Source: CAD feature listing. Evaluate the final solid. Frame: model axes, mm. A direction names the side the tool comes from. Round coordinates to 2 decimals unless told otherwise and drop trailing zeros. Loops run counter-clockwise (first coordinate to the right, second up) from the corner with the lowest first, then second, coordinate; pieces in that order, holes last. Notation, with made-up numbers: (13, 81) - (61, 81) arc R29 cw to (61, 112) - close; hole circle Ø11 at (-30, 53). An arc over 180 degrees is marked (long way). Write item = value, one per line. Start each with the question number.
from build123d import *

# Parameters (mm, degrees)
SKETCH1_R           = 2.5
BOSS_EXTRUDE1_DEPTH = 10
SKETCH2_R           = 7.5
BOSS_EXTRUDE2_DEPTH = 60
SKETCH3_R           = 2.5
CUT_EXTRUDE1_DEPTH  = 15


with BuildPart() as part:
    # Sketch1 → Boss-Extrude1 (new body)
    with BuildSketch(Plane.XY):
        with BuildLine():
            Line((2.5, 0), (37.6, 0))
            ThreePointArc((37.6, 0), (39.367766953, 0.732233047), (40.1, 2.5))
            Line((40.1, 2.5), (40.1, 37.6))
            ThreePointArc((40.1, 37.6), (39.367766953, 39.367766953), (37.6, 40.1))
            Line((37.6, 40.1), (2.5, 40.1))
            ThreePointArc((2.5, 40.1), (0.732233047, 39.367766953), (0, 37.6))
            Line((0, 37.6), (0, 2.5))
            ThreePointArc((0, 2.5), (0.732233047, 0.732233047), (2.5, 0))
        make_face()
        with Locations((6.75, 33.35)):
            Circle(SKETCH1_R, mode=Mode.SUBTRACT)
        with Locations((33.35, 6.75)):
            Circle(SKETCH1_R, mode=Mode.SUBTRACT)
    extrude(amount=BOSS_EXTRUDE1_DEPTH)

    # Sketch2 → Boss-Extrude2 (add)
    with BuildSketch(Plane.XY.offset(10)):
        with Locations((20.05, 20.05)):
            Circle(SKETCH2_R)
    extrude(amount=BOSS_EXTRUDE2_DEPTH)

    # Sketch3 → Cut-Extrude1 (cut)
    with BuildSketch(Plane.XY.offset(70)):
        with Locations((20.05, 20.05)):
            Circle(SKETCH3_R)
    extrude(amount=-CUT_EXTRUDE1_DEPTH, mode=Mode.SUBTRACT)


solid = part.part
(1) Cut plane C-C (z = 7). Output: boundary loops of the cut face in (x, y), and give its area (3 significant figures).
(2) Access query for faces 1 (the face through (29, 20, 10)), 2 (the face through (39.387, 39.348, 4.93)). Directions: +Z, -Z, +X, -X, +Y, -Y. A direction counts if a zero-diameter tool reaches every point of the face in a straight line with its end or side. Return the directions, or none.
(3) Cut plane D-D (x = 20.05). Output: boundary loops of the cut face in (y, z), and give its area (3 significant figures).
(4) Mould query, pull axis Y, two halves, no side actions, for faces 3 (the face through (26.98, 17.18, 39.58)), 4 (the face through (20, 20, 55)), 5 (the face through (0, 20, 5)), 6 (the face through (21.2, 17.83, 62.6)). Classes: +Y half, -Y half, draft (parallel to the pull), parting line (faces both ways), or undercut.
(5) Pin query (flat end, axial travel): P1, Ø1, axis at y = 18.5, z = 44, coming from the +X side; P2, Ø6, axis at y = 15, z = 62.5, coming from the -X side; P3, Ø8, axis at y = 18.5, z = 47.5, coming from the -X side. Return the tip coordinate at first contact, or that it passes through.
(6) Cut plane A-A (y = 33.35). Output: boundary loops of the cut face in (x, z).
(7) Cut plane B-B (x = 6.75). Output: boundary loops of the cut face in (y, z).
(8) Material intervals for line 1 along Y through (x, z) = (20, 60); line 2 along Y through (x, z) = (33.35, 3), sorted ascending. Write a range as from..to.
Solution:
q1.outline = (0, 2.5) arc R2.5 ccw to (2.5, 0) - (37.6, 0) arc R2.5 ccw to (40.1, 2.5) - (40.1, 37.6) arc R2.5 ccw to (37.6, 40.1) - (2.5, 40.1) arc R2.5 ccw to (0, 37.6) - close; hole circle Ø5 at (6.75, 33.35); hole circle Ø5 at (33.35, 6.75)
q1.area = 1,560 mm^2
q2.face_1 = +Z
q2.face_2 = +Z, -Z, +X, +Y
q3.outline = (0, 0) - (40.1, 0) - (40.1, 10) - (27.55, 10) - (27.55, 70) - (22.55, 70) - (22.55, 55) - (17.55, 55) - (17.55, 70) - (12.55, 70) - (12.55, 10) - (0, 10) - close
q3.area = 1,230 mm^2
q4.face_3 = parting line
q4.face_4 = undercut
q4.face_5 = draft
q4.face_6 = undercut
q5.P1 = 27.48
q5.P2 = 12.84
q5.P3 = 12.55
q6.outline = (0, 0) - (4.25, 0) - (4.25, 10) - (0, 10) - close; (9.25, 0) - (40.1, 0) - (40.1, 10) - (9.25, 10) - close
q7.outline = (0, 0) - (30.85, 0) - (30.85, 10) - (0, 10) - close; (35.85, 0) - (40.1, 0) - (40.1, 10) - (35.85, 10) - close
q8.line_1 = 12.55..17.55, 22.55..27.55
q8.line_2 = 0..4.25, 9.25..40.1
